Answer from the drawing. Dimensions are ordinates in mm from the lowest x, y and z of the part. A direction names the side the tool comes from. Coordinates: 2 decimals unless noted, no trailing zeros. Write each loop counter-clockwise with the first axis right and the second up, starting at its lowest first coordinate (ties: lowest second). Pieces come first, ordered by that corner, then holes. Notation, with made-up numbers: M 37.5,-0.75 L 94.5,-0.75 A11 ccw 94.5,7.25 Z; hole C -30,52 d4. An arc over 180 degrees is marked long. Put each result on its own line as item: value. Start each with the question number.
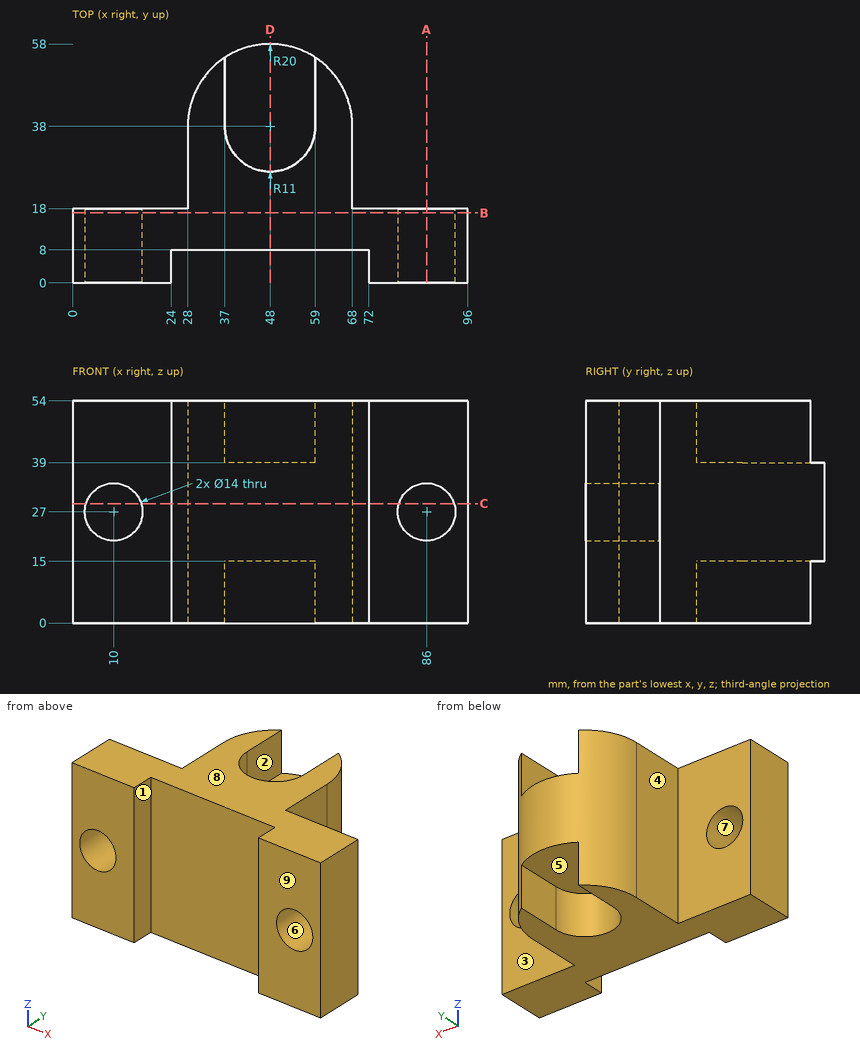
1) Straight lines are drawn through the part: probe 1 along Z at (x, y) = (10, 4); probe 2 along Z at (x, y) = (46, 31.5); probe 3 along X at (y, z) = (7, 37.5). For each, find the intervals that lie inside material, in ascending order.
2) For the marked faces 1, 2, 3, 4 and 5, determine the directions among +Z, -Z, +X, -X, +Y, -Y from which every point of the face is accessible in a straight line to the end or side of a thin tool.
3) A cutting plane is placed at A-A on x = 86. Write down the section's boundary in (y, z).
4) Given pin 1 Ø12 at (y, z) = (49.5, 8) entering from -X; pin 2 Ø18 at (x, z) = (10, 27) entering from +Y; pin 3 Ø14.5 at (x, z) = (43, 33.5) entering from -Y, each flat-ended and moving along its own axis, determine where each tip first touches the part or whether it passes through.
5) A cutting plane is placed at C-C on z = 29. Write down the section's boundary in (x, y), then the cut area to 3 significant figures.
6) Determine the mould class of the marked faces 6, 7, 8 and 9 for opening direction Z: +Z half, -Z half, draft (parallel to the pull), parting line (faces both ways), or undercut.
7) A cutting plane is placed at D-D on x = 48. Write down the section's boundary in (y, z).
8) A cutting plane is placed at B-B on y = 17. Write down the section's boundary in (x, z).
Answers follow:
1. probe 1: z = 0 to 20, 34 to 54
1. probe 2: z = 15 to 39
1. probe 3: x = 0 to 24, 72 to 96
2. face 1: +Z, -Z, -Y
2. face 2: +Z, +Y
2. face 3: +Z, -Z, +X, +Y
2. face 4: +Z, -Z, -X, +Y
2. face 5: -Z, +Y
3. outline: M 0,0 L 18,0 L 18,20 L 0,20 Z; M 0,34 L 18,34 L 18,54 L 0,54 Z
4. pin 1: stops at x = 28.77
4. pin 2: stops at y = 18
4. pin 3: stops at y = 8
5. outline: M 0,0 L 3.29,0 L 3.29,18 L 0,18 Z; M 16.71,0 L 24,0 L 24,8 L 72,8 L 72,0 L 79.29,0 L 79.29,18 L 68,18 L 68,38 A20 ccw 28,38 L 28,18 L 16.71,18 Z; M 92.71,0 L 96,0 L 96,18 L 92.71,18 Z
5. area: 2,290 mm²
6. face 6: undercut
6. face 7: undercut
6. face 8: +Z half
6. face 9: draft
7. outline: M 8,0 L 27,0 L 27,15 L 58,15 L 58,39 L 27,39 L 27,54 L 8,54 Z
8. outline: M 0,0 L 96,0 L 96,54 L 0,54 Z; hole C 10,27 d14; hole C 86,27 d14
